Could you check a few things on this model? Use its own coordinates, in mm. Face numbers are marked on the shaded views. A direction names the side the tool comes from. Round coordinates to 2 decimals unless told otherwise and drop trailing zeros. Write each loop counter-clockwise with the first axis right and the second up, starting at its lowest first coordinate (ties: lowest second). Pieces come first, ordered by that corner, then holes. Notation, with made-up numbers: (43, -2) -> (53, -2) arc R29 cw to (53, 28) -> close; hole circle Ø8 at (-37, 1.5). An arc over 180 degrees is marked (long way). Return JSON: item names as keys, results as strings.
from build123d import *

# Parameters (mm, degrees)
F1_DEPTH    = 70
F2_T        = -2.5
F3_T2_ANGLE = 48.492455887
F5_DEPTH    = 15
F6_T        = -2.5
F7_DEPTH    = 25


# Not quite as in the source:
# - a fillet or chamfer that OpenCascade refuses, or shapes differently, is made with other operations: its cross-section is extruded or revolved along the edge and cut away or added


with BuildPart() as f1:
    # F0 (on Top) → F1 (new body)
    with BuildSketch(Plane.XY):
        with BuildLine():
            ThreePointArc((-50, -141.4213562373), (-25.3652968089, -147.839783948), (0, -150))
            ThreePointArc((0, -150), (25.3652968089, -147.839783948), (50, -141.4213562373))
            Line((50, -141.4213562373), (50, -50))
            Line((50, -50), (0, -50))
            Line((0, -50), (-50, -50))
            Line((-50, -50), (-50, -141.4213562373))
        make_face()
    extrude(amount=F1_DEPTH)

    # F2
    f2_openings = [f1.faces().sort_by_distance(p)[0] for p in [
        (0, -98.620362, 70),
    ]]
    offset(amount=F2_T, openings=f2_openings)

    # F3: fillet of radius 5 on 1 edges, made by hand

    # F3_s1 → F3_t2 (revolve, cut)
    with BuildSketch(Plane(origin=(0, 0, 0), x_dir=(0, 0, 1), z_dir=(0.9117890812, 0.410658826, 0))):
        with BuildLine():
            ThreePointArc((65, 150), (68.5355339059, 148.5355339059), (70, 145))
            Line((70, 145), (70, 150))
            Line((70, 150), (65, 150))
        make_face()
    revolve(axis=Axis((0, 0, 70), (0, 0, -1)), revolution_arc=F3_T2_ANGLE, mode=Mode.SUBTRACT)

    # F4 (on face) → F5 (join)
    with BuildSketch(Plane(origin=(0, -50, 0), x_dir=(-1, 0, 0), z_dir=(0, 1, 0))):
        with BuildLine():
            ThreePointArc((32, 35.3235527873), (-22.627416998, 57.9509697853), (0, 3.3235527873))
            ThreePointArc((0, 3.3235527873), (22.627416998, 12.6961357893), (32, 35.3235527873))
        make_face()
    extrude(amount=F5_DEPTH)

    # F6
    f6_openings = [f1.faces().sort_by_distance(p)[0] for p in [
        (0, -35, 35.323553),
    ]]
    offset(amount=F6_T, openings=f6_openings, kind=Kind.INTERSECTION)

    # F7 (cut): a face of the model
    f7_faces = [f1.faces().sort_by_distance(p)[0] for p in [
        (0, -50, 35.3235527873),
    ]]
    extrude(f7_faces, amount=-F7_DEPTH, mode=Mode.SUBTRACT)


solid = f1.part
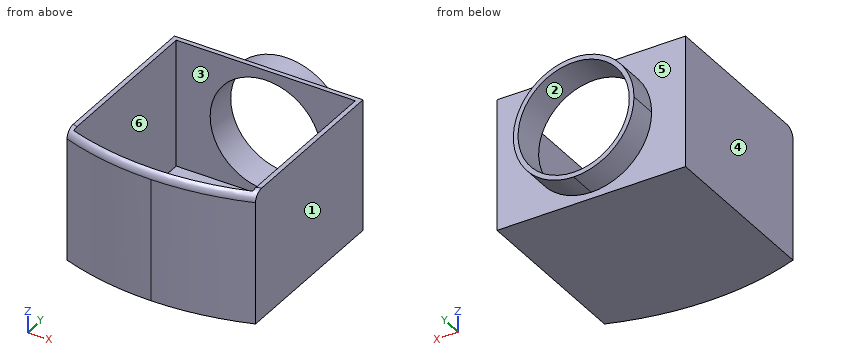
1) Will these pins go through, and if not, where does the flat tip stop? pin 1 Ø5 at (x, y) = (20, -124.5) entering from +Z; pin 2 Ø4 at (x, z) = (12, 22.5) entering from -Y; pin 3 Ø5 at (x, z) = (-34.5, 15) entering from -Y.
Return value:
{"pin 1": "z = 2.5", "pin 2": "y = -149.67", "pin 3": "y = -146.55"}
2) I want a section at C-C, the plane z = 29.5. Please give me the cut outline in (x, y).
Return value:
{"outline": "(-50, -141.42) arc R150 ccw to (50, -141.42) -> (50, -50) -> (31.47, -50) -> (31.47, -35) -> (28.92, -35) -> (28.92, -52.5) -> (47.5, -52.5) -> (47.5, -139.64) arc R147.5 cw to (-47.5, -139.64) -> (-47.5, -52.5) -> (-28.92, -52.5) -> (-28.92, -35) -> (-31.47, -35) -> (-31.47, -50) -> (-50, -50) -> close"}
3) For the marked faces 1, 2 and 3, which set-ups out of +Z, -Z, +X, -X, +Y, -Y let a thin tool reach every point of the face, with its end or its side?
Return value:
{"face 1": "+Z, -Z, +X, +Y, -Y", "face 2": "+Y", "face 3": "+Z"}
4) If I drill on probe 1 along X at (y, z) = (-71, 25); probe 2 along Z at (x, y) = (-0.5, -47); probe 3 along Y at (x, z) = (44.5, 58), over which ranges is the centre line in solid material (lowest first)? Write a range as [from, to].
Return value:
{"probe 1": "[-50, -47.5], [47.5, 50]", "probe 2": "[3.33, 5.83], [64.82, 67.32]", "probe 3": "[-143.25, -140.63], [-52.5, -50]"}
5) Thinking about a two-plate mould opening in Y: for the marked faces 4, 5 and 6, which applies, pulls with the +Y half, pulls with the -Y half, needs draft (parallel to the pull), parting line crosses it, or undercut?
Return value:
{"face 4": "needs draft", "face 5": "pulls with the +Y half", "face 6": "undercut"}
6) I want a section at B-B, the plane z = 41.5. Please give me the cut outline in (x, y).
Return value:
{"outline": "(-50, -141.42) arc R150 ccw to (50, -141.42) -> (50, -50) -> (31.4, -50) -> (31.4, -35) -> (28.85, -35) -> (28.85, -52.5) -> (47.5, -52.5) -> (47.5, -139.64) arc R147.5 cw to (-47.5, -139.64) -> (-47.5, -52.5) -> (-28.85, -52.5) -> (-28.85, -35) -> (-31.4, -35) -> (-31.4, -50) -> (-50, -50) -> close"}
7) I want a section at A-A, the plane y = -55. Please give me the cut outline in (x, z).
Return value:
{"outline": "(-50, 0) -> (50, 0) -> (50, 70) -> (47.5, 70) -> (47.5, 2.5) -> (-47.5, 2.5) -> (-47.5, 70) -> (-50, 70) -> close"}
